The drawing under review shows one solid part. Ordinate dimensions are in mm from its lowest x, y, z. Give positions to 0.01 mm unless a question says otherwise; leave off trailing zeros. Order: outer loops, then holes, each group sorted by start corner. A loop starts at its lowest first (then second) coordinate and runs counter-clockwise, first axis right, second up. Notation, with made-up numbers: (8, -23) - (44, -23) arc R12 ccw to (44, -14) - close; hole circle Ø4 at (-35.75, 73.5). An arc over 180 degrees is marked (long way). Write item = value, one per line. Start each with the question number.
1. We need section C-C, the plane y = 0.5. Give the boundary of the cut face in (x, z) (3 decimals), and give its area (3 significant figures).
2. We need section D-D, the plane z = 29.21. Give the boundary of the cut face in (x, y) (3 decimals), and give its area (3 significant figures).
3. We need section A-A, the plane z = 16.51. Give the boundary of the cut face in (x, y) (3 decimals), and give its area (3 significant figures).
4. Wall thickness on probe 1 along Z at (x, y) = (34.29, 0.2) (3 decimals); probe 2 along Z at (x, y) = (35, 0.3); probe 3 along X at (y, z) = (0.4, 5): over which ranges is each line inside the solid? List them lowest first.
5. We need section B-B, the plane x = 19.05. Give the boundary of the cut face in (y, z) (3 decimals).
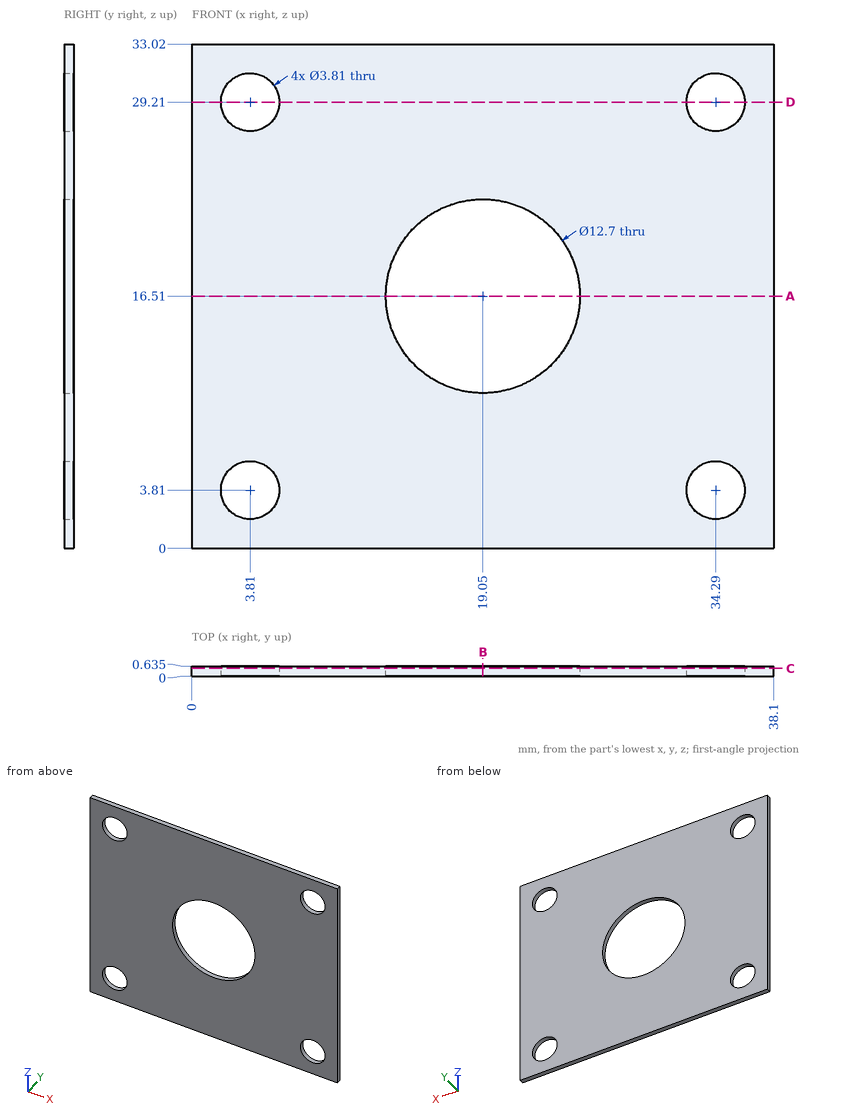
Model answer:
q1.outline = (0, 0) - (38.1, 0) - (38.1, 33.02) - (0, 33.02) - close; hole circle Ø3.81 at (3.81, 3.81); hole circle Ø3.81 at (3.81, 29.21); hole circle Ø12.7 at (19.05, 16.51); hole circle Ø3.81 at (34.29, 3.81); hole circle Ø3.81 at (34.29, 29.21)
q1.area = 1,090 mm2
q2.outline = (0, 0) - (1.905, 0) - (1.905, 0.635) - (0, 0.635) - close; (5.715, 0) - (32.385, 0) - (32.385, 0.635) - (5.715, 0.635) - close; (36.195, 0) - (38.1, 0) - (38.1, 0.635) - (36.195, 0.635) - close
q2.area = 19.4 mm2
q3.outline = (0, 0) - (12.7, 0) - (12.7, 0.635) - (0, 0.635) - close; (25.4, 0) - (38.1, 0) - (38.1, 0.635) - (25.4, 0.635) - close
q3.area = 16.1 mm2
q4.probe_1 = 0 to 1.905, 5.715 to 27.305, 31.115 to 33.02
q4.probe_2 = 0 to 2.04, 5.58 to 27.44, 30.98 to 33.02
q4.probe_3 = 0 to 2.32, 5.3 to 32.8, 35.78 to 38.1
q5.outline = (0, 0) - (0.635, 0) - (0.635, 10.16) - (0, 10.16) - close; (0, 22.86) - (0.635, 22.86) - (0.635, 33.02) - (0, 33.02) - close
